Read the model definition and answer for the solid it produces. Units are mm, in the model's axes. A direction names the side the tool comes from. Round coordinates to 2 decimals unless told otherwise and drop trailing zeros. Write each loop counter-clockwise with the first axis right and the second up, starting at its lowest first coordinate (ties: lowest second). Pieces come first, ordered by that corner, then holes. Notation, with made-up numbers: (28.25, 23.5) -> (63.25, 23.5) arc R18 ccw to (63.25, 57.5) -> close; hole circle Ø3 at (64.5, -18). An arc over 180 degrees is marked (long way). Return JSON: item names as keys, results as strings. Group by question number.
(1) A cutting plane is placed at B-B on x = -174.5. Give the vertices of the cut face in (y, z), then the cut area to 3 significant figures.
(2) The mould has two halves that part along X. Classify faces 4 (the cylindrical face through (8.81, -3.24, 12.67)), 5 (the flat face through (-185.39, 6, 18)), 6 (the flat face through (-93, 10.047, 12)), 7 (the cylindrical face through (-175.453, -0.352, 17.605)): released by +X, released by -X, zero draft, split by the parting line, or undercut.
(3) Straight lines are drawn through the part: line 1 (X direction, y = -1.5, z = 17.5); line 2 (X direction, y = 2.5, z = 24); line 3 (X direction, y = -3, z = 17.5). For each, find the intervals that lie inside material, in ascending order.
(4) A cutting plane is placed at A-A on z = 13.5. Give the vertices of the cut face in (x, y).
(5) Given pin 1 (2.5 mm diameter, centred on x = -183.5, y = -3, fed in from -Z); pin 2 (5.5 mm diameter, centred on x = -181, z = 21, fed in from +Y); pin 3 (1 mm diameter, centred on y = 5.5, z = 5, fed in from +X), each flat-ended and moving along its own axis, determine where each tip first touches the part or whether it passes through.
(6) For faces 1 (the flat face through (-175, 3, 2)), 2 (the flat face through (-91, 3, 25)), 3 (the flat face through (-180, 2.547, 18)), determine the directions among +Z, -Z, +X, -X, +Y, -Y from which every point of the face is accessible in a straight line to the end or side of a thin tool.
```python
from build123d import *

# Parameters (mm, degrees)
IZIM1_W                     = 200
IZIM1_H                     = 15
Y_KSEKLIK_EKSTR_ZYON1_DEPTH = 25
RADYUS1_R                   = 6
IZIM3_R                     = 2.9
KES_EKSTR_ZYON2_DEPTH       = 1
KES_EKSTR_ZYON2_DEPTH_BACK  = 15
KES_EKSTR_ZYON3_DEPTH       = 10
IZIM6_R                     = 1.45
KES_EKSTR_ZYON4_DEPTH       = 2
IZIM8_W                     = 20
IZIM8_H                     = 7.5
KES_EKSTR_ZYON6_DEPTH       = 15
IZIM9_R                     = 1.5
KES_EKSTR_ZYON7_DEPTH       = 15
RADYUS2_R                   = 0.5


with BuildPart() as part:
    # Çizim1 → Yükseklik-Ekstrüzyon1 (new body)
    with BuildSketch(Plane.XY):
        with Locations((-89.389671362, 2.546948357)):
            Rectangle(IZIM1_W, IZIM1_H)
    extrude(amount=Y_KSEKLIK_EKSTR_ZYON1_DEPTH)

    # Radyus1
    radyus1_edges = [part.edges().sort_by_distance(p)[0] for p in [
        (10.610328638, -4.953051643, 12.5),
        (10.610328638, 10.046948357, 12.5),
    ]]
    fillet(radyus1_edges, radius=RADYUS1_R)

    # Çizim3 → Kes-Ekstrüzyon2 (cut, two sides)
    with BuildSketch(Plane.XY.offset(25)) as kes_ekstr_zyon2_sk:
        with Locations((-175.389671362, 2.546948357)):
            Circle(IZIM3_R)
    extrude(amount=KES_EKSTR_ZYON2_DEPTH, mode=Mode.SUBTRACT)
    extrude(kes_ekstr_zyon2_sk.sketch, amount=-KES_EKSTR_ZYON2_DEPTH_BACK, mode=Mode.SUBTRACT)

    # Çizim4 → Kes-Ekstrüzyon3 (cut)
    with BuildSketch(Plane(origin=(0, 0, 0), x_dir=(-1, 0, 0), z_dir=(0, 0, -1))):
        with BuildLine():
            ThreePointArc((167.639671362, -0.633051643), (166.614366529, -3.108356476), (169.089671362, -2.083051643))
            Line((169.089671362, -2.083051643), (167.639671362, -2.083051643))
            Line((167.639671362, -2.083051643), (167.639671362, -0.633051643))
        make_face()
        with BuildLine():
            Line((167.639671362, -2.083051643), (169.089671362, -2.083051643))
            ThreePointArc((169.089671362, -2.083051643), (168.664976194, -1.05774681), (167.639671362, -0.633051643))
            Line((167.639671362, -0.633051643), (167.639671362, -2.083051643))
        make_face()
        with BuildLine():
            ThreePointArc((184.589671362, -2.083051643), (184.164976194, -1.05774681), (183.139671362, -0.633051643))
            Line((183.139671362, -0.633051643), (183.139671362, -2.083051643))
            Line((183.139671362, -2.083051643), (181.689671362, -2.083051643))
            ThreePointArc((181.689671362, -2.083051643), (183.139671362, -3.533051643), (184.589671362, -2.083051643))
        make_face()
        with BuildLine():
            Line((183.139671362, -2.083051643), (183.139671362, -0.633051643))
            ThreePointArc((183.139671362, -0.633051643), (182.114366529, -1.05774681), (181.689671362, -2.083051643))
            Line((181.689671362, -2.083051643), (183.139671362, -2.083051643))
        make_face()
    extrude(amount=-KES_EKSTR_ZYON3_DEPTH, mode=Mode.SUBTRACT)

    # Çizim6 → Kes-Ekstrüzyon4 (cut)
    with BuildSketch(Plane(origin=(0, 0, 0), x_dir=(-1, 0, 0), z_dir=(0, 0, -1))):
        Polygon((185.839671362, -4.953051643), (185.839671362, -2.083051643), (185.839671362, 10.046948357), (165.238795476, 10.046948357), (164.839671362, 10.046948357), (164.839671362, -4.953051643), align=None)
        with Locations((167.639671362, -2.083051643)):
            Circle(IZIM6_R, mode=Mode.SUBTRACT)
        with Locations((183.139671362, -2.083051643)):
            Circle(IZIM6_R, mode=Mode.SUBTRACT)
    extrude(amount=-KES_EKSTR_ZYON4_DEPTH, mode=Mode.SUBTRACT)

    # Çizim8 → Kes-Ekstrüzyon6 (cut)
    with BuildSketch(Plane.XY.offset(25)):
        with Locations((-175.389671362, 6.296948357)):
            Rectangle(IZIM8_W, IZIM8_H)
    extrude(amount=-KES_EKSTR_ZYON6_DEPTH, mode=Mode.SUBTRACT)

    # Çizim9 → Kes-Ekstrüzyon7 (cut)
    with BuildSketch(Plane(origin=(0, 2.546948357, 0), x_dir=(1, 0, 0), z_dir=(0, 1, 0))):
        with Locations((-168.889671362, -17.5)):
            Circle(IZIM9_R)
        with Locations((-181.889671362, -17.5)):
            Circle(IZIM9_R)
    extrude(amount=-KES_EKSTR_ZYON7_DEPTH, mode=Mode.SUBTRACT)

    # Radyus2
    radyus2_edges = [part.edges().sort_by_distance(p)[0] for p in [
        (-189.389671362, 2.546948357, 25),
        (-92.389671362, -4.953051643, 25),
        (10.610328638, 2.546948357, 0),
        (10.610328638, 2.546948357, 25),
        (-80.114671362, 10.046948357, 0),
        (8.852969326, 8.289589044, 0),
        (8.852969326, -3.19569233, 0),
        (-80.389671362, 10.046948357, 25),
        (8.852969326, 8.289589044, 25),
        (8.852969326, -3.19569233, 25),
        (-80.114671362, -4.953051643, 0),
        (-187.614671362, 10.046948357, 0),
        (-187.614671362, -4.953051643, 0),
        (-185.839671362, 2.546948357, 2),
        (-189.389671362, 2.546948357, 0),
        (-164.839671362, 2.546948357, 2),
        (-187.389671362, 10.046948357, 25),
        (-189.389671362, -4.953051643, 12.5),
        (-189.389671362, 10.046948357, 12.5),
    ]]
    fillet(radyus2_edges, radius=RADYUS2_R)


solid = part.part
```
Checks:
{
 "1": {"outline": "(-4.95, 2) -> (10.05, 2) -> (10.05, 10) -> (-0.21, 10) -> (-0.21, 25) -> (-4.45, 25) arc R0.5 ccw to (-4.95, 24.5) -> close", "area": "191 mm^2"},
 "2": {"face 4": "released by +X", "face 5": "undercut", "face 6": "zero draft", "face 7": "undercut"},
 "3": {"line 1": "x = -189.39 to -183.39, -180.39 to -170.39, -167.39 to 10.04", "line 2": "x = -189.39 to -178.29, -172.49 to 10.61", "line 3": "x = -189.39 to -183.39, -180.39 to -170.39, -167.39 to 9.04"},
 "4": {"outline": "(-189.39, -4.45) arc R0.5 ccw to (-188.89, -4.95) -> (4.61, -4.95) arc R6 ccw to (10.61, 1.05) -> (10.61, 4.05) arc R6 ccw to (4.61, 10.05) -> (-165.39, 10.05) -> (-165.39, 2.55) -> (-172.49, 2.55) arc R2.9 cw to (-178.29, 2.55) -> (-185.39, 2.55) -> (-185.39, 10.05) -> (-188.89, 10.05) arc R0.5 ccw to (-189.39, 9.55) -> close"},
 "5": {"pin 1": "stops at z = 2", "pin 2": "stops at y = 2.55", "pin 3": "stops at x = 10.53"},
 "6": {"face 1": "-Z, +Y, -Y", "face 2": "+Z, +X, -X, +Y, -Y", "face 3": "+Z, +Y"}
}
